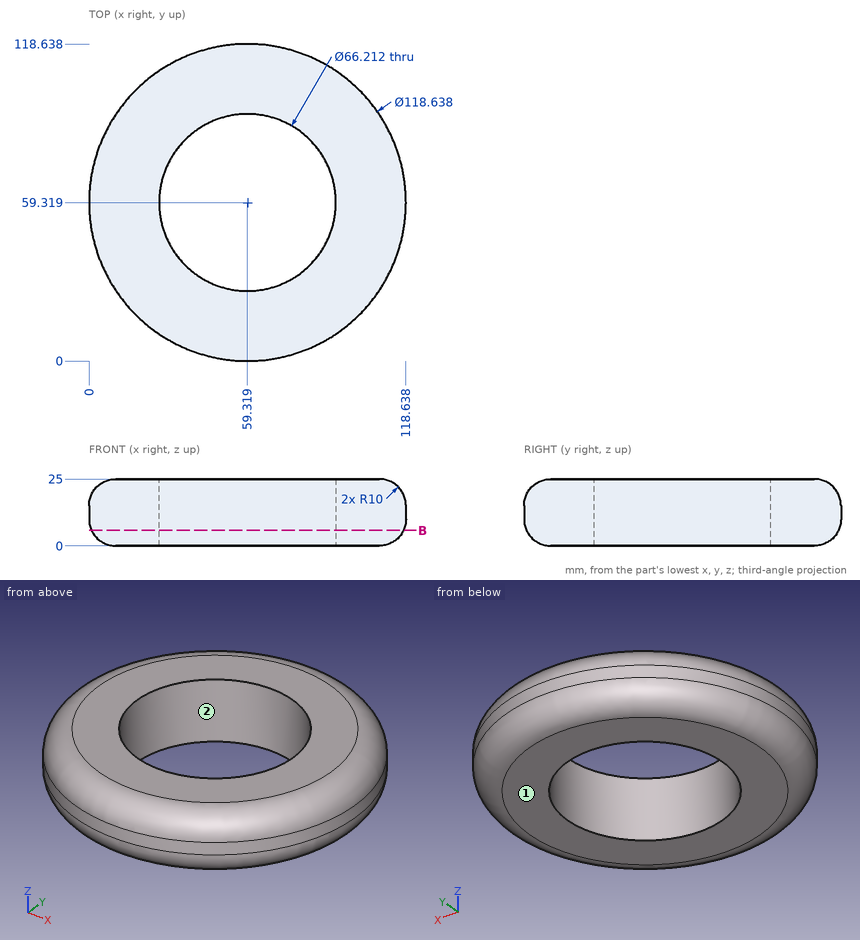
For this review, use the dimensioned drawing (mm, ordinates from the lowest corner) and the shaded views. Coordinates: 2 decimals unless noted, no trailing zeros. Write each loop counter-clockwise with the first axis right and the second up, starting at its lowest first coordinate (ties: lowest second). Pieces come first, ordered by that corner, then holes. Notation, with made-up numbers: (85, -28.5) -> (132, -28.5) arc R18 ccw to (132, 6.5) -> close; hole circle Ø4 at (5.25, 50.25). An arc over 180 degrees is marked (long way). Write each question's results on one line, items separated by ' | '. Start each with the question number.
(1) Take a section at B-B on z = 5.75. Write out the cut boundary in (x, y) (1 decimal).
(2) Clearance check with flat-ended pins moving along their axes: P1, Ø5, axis at y = 70, z = 4, coming from the +X side; P2, Ø1.5, axis at x = 58, z = 8.5, coming from the -Y side; P3, Ø6, axis at y = 53.5, z = 5.5, coming from the +X side. State where each tip first meets the part, or that it passes through.
(3) For line 1 along X through (y, z) = (70.5, 5.75); line 2 along Y through (x, z) = (78.5, 21.25) (1 decimal); line 3 along X through (y, z) = (29.5, 21.5) (1 decimal), list the stretches that pass through material, from the lowest coordinate up. Write a range as from..to.
(4) The part is to be moulded in two halves that separate along Y. For the marked faces 1 and 2, say which applies: pulls with the +Y half, pulls with the -Y half, needs draft (parallel to the pull), parting line crosses it, or undercut.
Results found:
1) outline: circle Ø116.7 at (59.3, 59.3); hole circle Ø66.2 at (59.3, 59.3)
2) P1: stops at x = 117.12 | P2: stops at y = 0.04 | P3: stops at x = 118.3
3) line 1: x = 2.03..28.16, 90.48..116.61 | line 2: y = 5.5..32.3, 86.3..113.1 | line 3: x = 10.8..44.9, 73.7..107.8
4) face 1: needs draft | face 2: undercut
